```python
from build123d import *

# Parameters (mm, degrees)
SKETCH1_R           = 31.75
BOSS_EXTRUDE1_DEPTH = 7.62
BOSS_EXTRUDE2_START = -7.62
SKETCH2_W           = 63.5
SKETCH2_H           = 101.6
BOSS_EXTRUDE2_DEPTH = 7.62
SKETCH4_W           = 25.4
SKETCH4_H           = 71.12
CUT_EXTRUDE2_DEPTH  = 107.717790925
FILLET1_R           = 28.575
SKETCH6_W           = 7.62
SKETCH6_H           = 19.05
BOSS_EXTRUDE3_DEPTH = 63.5
SKETCH5_R           = 2.032
CUT_EXTRUDE3_DEPTH  = 128.22839463
SKETCH3_R           = 24.384
CUT_EXTRUDE1_DEPTH  = 7.62
SKETCH7_W           = 12.7
SKETCH7_H           = 7.62
CUT_EXTRUDE4_DEPTH  = 124.529943334


with BuildPart() as part:
    # Sketch1 → Boss-Extrude1 (new body)
    with BuildSketch(Plane.XY):
        with Locations(Location((0, 0, 0), (0, 0, 180))):
            Circle(SKETCH1_R)
    extrude(amount=BOSS_EXTRUDE1_DEPTH)

    # Sketch2 → Boss-Extrude2 (add)
    with BuildSketch(Plane.XY.offset(7.62).offset(BOSS_EXTRUDE2_START)):
        with Locations((0, -50.8)):
            Rectangle(SKETCH2_W, SKETCH2_H)
    extrude(amount=BOSS_EXTRUDE2_DEPTH)

    # Sketch4 → Cut-Extrude2 (cut, through all)
    with BuildSketch(Plane.XY.offset(7.62)):
        with Locations((-19.05, -66.04)):
            Rectangle(SKETCH4_W, SKETCH4_H)
        with Locations((19.05, -66.04)):
            Rectangle(SKETCH4_W, SKETCH4_H)
    extrude(amount=-CUT_EXTRUDE2_DEPTH, mode=Mode.SUBTRACT)

    # Fillet1
    # the kernel refuses this fillet: 28.575 mm, written as the material it takes off along each edge
    with BuildSketch(Plane(origin=(31.75, -30.48, 78.615158286), x_dir=(0, 1, 0), z_dir=(0, 0, -1))) as fillet1_piece_1:
        with BuildLine():
            CenterArc((28.398063314, -28.575), FILLET1_R, 90, 83.620629792)
            Line((0, -25.4), (-0.567961266, -25.3365))
            ThreePointArc((-0.567961266, -25.3365), (-0.5715, -12.7), (-0.5715, 0))
            Line((-0.5715, 0), (0, 0.5715))
            Line((0, 0.5715), (28.398063314, 0.5715))
            Line((28.398063314, 0.5715), (28.398063314, 0))
        make_face()
    extrude(amount=149.610316571, mode=Mode.SUBTRACT)
    with BuildSketch(Plane(origin=(-31.75, -30.48, 78.615158286), x_dir=(1, 0, 0), z_dir=(0, 0, -1))) as fillet1_piece_2:
        with BuildLine():
            CenterArc((28.575, -28.398063314), FILLET1_R, 96.379370208, 83.620629792)
            Line((0, -28.398063314), (-0.5715, -28.398063314))
            Line((-0.5715, -28.398063314), (-0.5715, 0))
            Line((-0.5715, 0), (0, 0.5715))
            ThreePointArc((0, 0.5715), (12.7, 0.5715), (25.3365, 0.567961266))
            Line((25.3365, 0.567961266), (25.4, 0))
        make_face()
    extrude(amount=149.610316571, mode=Mode.SUBTRACT)

    # Sketch6 → Boss-Extrude3 (add)
    with BuildSketch(Plane.ZY.offset(6.35)):
        with Locations((3.81, -20.955)):
            Rectangle(SKETCH6_W, SKETCH6_H)
    boss_extrude3 = extrude(amount=BOSS_EXTRUDE3_DEPTH)

    # Mirror1: Boss-Extrude3 across plane
    add(boss_extrude3.mirror(Plane(origin=(0, 0, 0), x_dir=(0, 0, 1), z_dir=(1, 0, 0))))

    # Sketch5 → Cut-Extrude3 (cut, through all)
    with BuildSketch(Plane.ZY.offset(6.35)):
        with Locations((3.81, -95.25)):
            Circle(SKETCH5_R)
    extrude(amount=-CUT_EXTRUDE3_DEPTH, mode=Mode.SUBTRACT)

    # Sketch3 → Cut-Extrude1 (cut)
    with BuildSketch(Plane.XY.offset(7.62)):
        Circle(SKETCH3_R)
    extrude(amount=-CUT_EXTRUDE1_DEPTH, mode=Mode.SUBTRACT)

    # Sketch7 → Cut-Extrude4 (cut, through all)
    with BuildSketch(Plane.XY.offset(7.62)):
        with Locations((-48.26, -22.86)):
            Rectangle(SKETCH7_W, SKETCH7_H)
    cut_extrude4 = extrude(amount=-CUT_EXTRUDE4_DEPTH, mode=Mode.SUBTRACT)

    # Mirror2: Cut-Extrude4 across plane
    add(cut_extrude4.mirror(Plane(origin=(0, 0, 0), x_dir=(0, 0, 1), z_dir=(1, 0, 0))), mode=Mode.SUBTRACT)


solid = part.part
```
Work out the finished part from the listing and answer in its coordinate system (mm). A direction names the side the tool comes from. Give positions to 0.01 mm unless a question says otherwise; leave off trailing zeros. Loops run counter-clockwise (first coordinate to the right, second up) from the corner with the lowest first, then second, coordinate; pieces in that order, holes last. Notation, with made-up numbers: (26, -37) -> (83, -37) arc R7 cw to (83, -32) -> close; hole circle Ø1 at (86, 41.25). An arc over 180 degrees is marked (long way). Write item = value, one per line. Start each with the question number.
(1) Find the intervals of material crossed by probe 1 along Y at (x, z) = (-0.5, 3.81); probe 2 along Y at (x, z) = (0.5, 3); probe 3 along Y at (x, z) = (-44, 5.25), in increasing order. Write a range as from..to.
(2) Find section B-B on x = 0. Give the vertices of the cut face in (y, z), and give its area (3 significant figures).
(3) Find section C-C on x = -47.5. Give the vertices of the cut face in (y, z).
(4) Find section A-A on z = 3.81. Give the vertices of the cut face in (x, y) (3 decimals), and give its area (3 significant figures).
(5) Given pin 1 Ø2.5 at (x, z) = (-48, 3) entering from +Y; pin 2 Ø1.5 at (y, z) = (-53, 2.5) entering from +X; pin 3 Ø2.5 at (y, z) = (-49.5, 2.5) entering from -X, each flat-ended and moving along its own axis, determine where each tip first touches the part or whether it passes through.
(6) Which of the six approach directions +Z, -Z, +X, -X, +Y, -Y give full straight-line access (tool end or side, diameter ignored) to faces 4 (the flat face through (6.35, -67, 4)), 5 (the flat face through (-48, -26.67, 4)), 6 (the flat face through (-6.35, -67, 4)), 7 (the cylindrical face through (0.698, 31.742, 3.757))?
(7) Find section D-D on y = -95.25. Give the vertices of the cut face in (x, z), and give its area (3 significant figures).
(8) The mould has two halves that part along Z. Classify faces 1 (the cylindrical face through (-0.089, -93.235, 3.545)), 2 (the flat face through (0, -30, 0)), 3 (the cylindrical face through (-3.174, 24.177, 3.863)): +Z half, -Z half, draft (parallel to the pull), parting line (faces both ways), or undercut.
From the geometry:
q1.probe_1 = -101.6..-97.28, -93.22..-24.38, 24.38..31.75
q1.probe_2 = -101.6..-97.11, -93.39..-24.38, 24.38..31.75
q1.probe_3 = -30.48..-26.67, -19.05..-11.43
q2.outline = (-101.6, 0) -> (-24.38, 0) -> (-24.38, 7.62) -> (-101.6, 7.62) -> close; (24.38, 0) -> (31.75, 0) -> (31.75, 7.62) -> (24.38, 7.62) -> close; hole circle Ø4.06 at (-95.25, 3.81)
q2.area = 632 mm^2
q3.outline = (-30.48, 0) -> (-26.67, 0) -> (-26.67, 7.62) -> (-30.48, 7.62) -> close; (-19.05, 0) -> (-11.43, 0) -> (-11.43, 7.62) -> (-19.05, 7.62) -> close
q4.outline = (-69.85, -30.48) -> (-6.35, -30.48) -> (-6.35, -93.218) -> (6.35, -93.218) -> (6.35, -30.48) -> (69.85, -30.48) -> (69.85, -11.43) -> (30.178, -11.43) arc R28.575 ccw to (31.75, -2.082) -> (31.75, 0) arc R31.75 ccw to (-31.75, 0) -> (-31.75, -2.082) arc R28.575 ccw to (-30.178, -11.43) -> (-69.85, -11.43) -> close; (-6.35, -101.6) -> (6.35, -101.6) -> (6.35, -97.282) -> (-6.35, -97.282) -> close; hole (-54.61, -26.67) -> (-41.91, -26.67) -> (-41.91, -19.05) -> (-54.61, -19.05) -> close; hole circle Ø48.768 at (0, 0); hole (41.91, -26.67) -> (54.61, -26.67) -> (54.61, -19.05) -> (41.91, -19.05) -> close
q4.area = 3,750 mm^2
q5.pin_1 = -11.43
q5.pin_2 = 6.35
q5.pin_3 = -6.35
q6.face_4 = +Z, -Z, +X, -Y
q6.face_5 = +Z, -Z
q6.face_6 = +Z, -Z, -X, -Y
q6.face_7 = +Z, -Z, +Y
q7.outline = (-6.35, 0) -> (6.35, 0) -> (6.35, 1.78) -> (-6.35, 1.78) -> close; (-6.35, 5.84) -> (6.35, 5.84) -> (6.35, 7.62) -> (-6.35, 7.62) -> close
q7.area = 45.2 mm^2
q8.face_1 = undercut
q8.face_2 = -Z half
q8.face_3 = draft
